from build123d import *

# Parameters (mm, degrees)
INSIDEBOREF_R = 0.5


with BuildPart() as part:
    # MainBodyS → MainBody (revolve)
    with BuildSketch(Plane.XY, mode=Mode.PRIVATE) as mainbody_sk:
        Polygon((0, 15.8), (4.75, 15.8), (5.05, 1), (6.5, 1), (6.5, 0), (4.070064849, 0), (3.784254039, 14.1), (0, 14.1), align=None)
    revolve(mainbody_sk.sketch.rotate(Axis((0, 0, 0), (0, 1, 0)), 90), axis=Axis((0, 0, 0), (0, 1, 0)))

    # InsertBodyS → InsertBody (revolve)
    with BuildSketch(Plane.XY, mode=Mode.PRIVATE) as insertbody_sk:
        Polygon((5.02972973, 2), (6.1, 2), (6.1, 1), (5.05, 1), align=None)
    revolve(insertbody_sk.sketch.rotate(Axis((0, 1, 0), (0, -1, 0)), 270), axis=Axis((0, 1, 0), (0, -1, 0)))

    # InsideBoreF
    insideboref_edges = [part.edges().sort_by_distance(p)[0] for p in [
        (0, 0, 4.070064849),
    ]]
    fillet(insideboref_edges, radius=INSIDEBOREF_R)


solid = part.part
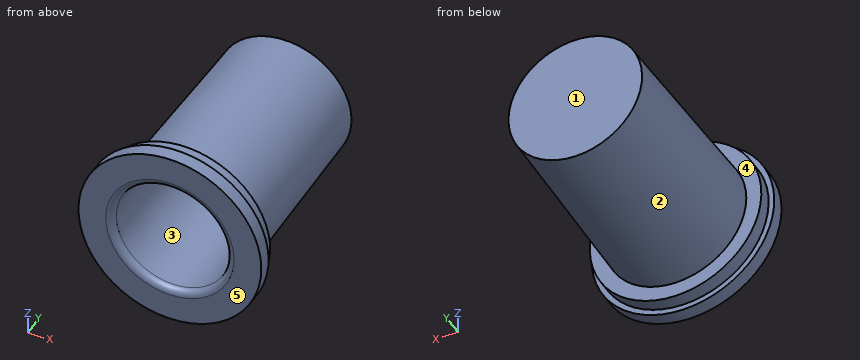
Geometry: final body of the model. Coordinates: model frame, mm. Face numbers are marked on the shaded views. A direction names the side the tool comes from. Give positions to 0.01 mm unless a question says otherwise; leave off trailing zeros. Order: outer loops, then holes, each group sorted by start corner. A loop starts at its lowest first (then second) coordinate and runs counter-clockwise, first axis right, second up. Notation, with made-up numbers: (-19, 32) -> (-2, 32) arc R23 cw to (-2, 48) -> close; hole circle Ø9 at (43.5, 79.25). An arc over 180 degrees is marked (long way). Answer as a JSON object with one key per item and string values.
Q1. Material intervals for probe 1 along Z at (x, y) = (-1, 9.75); probe 2 along Z at (x, y) = (1.5, 4.5); probe 3 along Y at (x, z) = (0.5, -2), sorted ascending.
Entries:
{"probe 1": "z = -4.77 to -3.74, 3.74 to 4.77", "probe 2": "z = -4.75 to -3.69, 3.69 to 4.75", "probe 3": "y = 14.1 to 15.8"}
Q2. Section B-B (x = 0). Output: boundary loops of the cut face in (y, z).
Entries:
{"outline": "(0, -6.5) -> (1, -6.5) -> (1, -6.1) -> (2, -6.1) -> (2, -5.03) -> (15.8, -4.75) -> (15.8, 4.75) -> (2, 5.03) -> (2, 6.1) -> (1, 6.1) -> (1, 6.5) -> (0, 6.5) -> (0, 4.56) arc R0.5 ccw to (0.49, 4.06) -> (14.1, 3.78) -> (14.1, -3.78) -> (0.49, -4.06) arc R0.5 ccw to (0, -4.56) -> close"}
Q3. Section D-D (x = 5.25). Output: boundary loops of the cut face in (y, z), plus the area to 3 significant figures.
Entries:
{"outline": "(0, -3.83) -> (1, -3.83) -> (1, -3.11) -> (2, -3.11) -> (2, 3.11) -> (1, 3.11) -> (1, 3.83) -> (0, 3.83) -> close", "area": "13.9 mm^2"}
Q4. Section C-C (y = 9). Output: boundary loops of the cut face in (x, z).
Entries:
{"outline": "circle Ø9.78 at (0, 0); hole circle Ø7.78 at (0, 0)"}
Q5. First-contact query: pin 1 (2 mm diameter, centred on y = 9.5, z = 3.5, fed in from +X); pin 2 (4 mm diameter, centred on x = 0, y = 12.5, fed in from -Z). Flat tips, straight axial feed; report the tip coordinate or a pass-through.
Entries:
{"pin 1": "stops at x = 4.19", "pin 2": "stops at z = -4.86"}
Q6. Section A-A (z = 0). Output: boundary loops of the cut face in (x, y), plus the area to 3 significant figures.
Entries:
{"outline": "(-6.5, 0) -> (-4.56, 0) arc R0.5 ccw to (-4.06, 0.49) -> (-3.78, 14.1) -> (3.78, 14.1) -> (4.06, 0.49) arc R0.5 ccw to (4.56, 0) -> (6.5, 0) -> (6.5, 1) -> (6.1, 1) -> (6.1, 2) -> (5.03, 2) -> (4.75, 15.8) -> (-4.75, 15.8) -> (-5.03, 2) -> (-6.1, 2) -> (-6.1, 1) -> (-6.5, 1) -> close", "area": "49.3 mm^2"}
Q7. Access query for the marked faces 4 and 5. Directions: +Z, -Z, +X, -X, +Y, -Y. A direction counts if a zero-diameter tool reaches every point of the face in a straight line with its end or side. Return the directions, or none.
Entries:
{"face 4": "+Y", "face 5": "+Z, -Z, +X, -X, -Y"}
Q8. Draft query along X for the marked faces 1, 2 and 3. Return one class per face: released by +X, released by -X, zero draft, split by the parting line, or undercut.
Entries:
{"face 1": "zero draft", "face 2": "split by the parting line", "face 3": "undercut"}
